Autodesk Inventor part; units mm, degrees
ref_plane "YZ Plane" through (0, 0, 0) normal (1, 0, 0) x (0, 1, 0)
ref_plane "XZ Plane" through (0, 0, 0) normal (0, 1, 0) x (-1, 0, 0)
ref_plane "XY Plane" through (0, 0, 0) normal (0, 0, 1) x (1, 0, 0)
sketch "Эскиз1" plane through (0, 0, 0) normal (0, 0, 1) x (1, 0, 0)
  line L0 (-54, -14) -> (54, -14)
  line L1 (54, -14) -> (54, 14)
  line L2 (54, 14) -> (-54, 14)
  line L3 (-54, 14) -> (-54, -14)
  line L4 (-54, -14) -> (54, 14) construction
  line L5 (54, -14) -> (-54, 14) construction
  point P0 (0, 0)
  dimension "d0" = 108
  dimension "d1" = 28
extrude "Выдавливание1" add sketch "Эскиз1" along normal blind 27.5
sketch "Эскиз2" plane through (0, 0, 27.5) normal (0, 0, 1) x (1, 0, 0)
  line L0 (-51, -11) -> (51, -11)
  line L1 (51, -11) -> (51, 11)
  line L2 (51, 11) -> (-51, 11)
  line L3 (-51, 11) -> (-51, -11)
  line L4 (-51, -11) -> (51, 11) construction
  line L5 (51, -11) -> (-51, 11) construction
  line L6 (54, 14) -> (-54, 14)
  line L7 (54, -14) -> (54, 14)
  point P0 (0, 0)
  dimension "d4" = 3
  dimension "d5" = 3
extrude "Выдавливание2" cut sketch "Эскиз2" against normal blind 24.5
sketch "Эскиз3" plane through (54, -14, 0) normal (1, 0, 0) x (0, 0, -1)
  line L0 (0, 28) -> (-27.5, 28)
  line L1 (0, 0) -> (-27.5, 0)
  line L2 (-27.5, 28) -> (-26, 28)
  line L3 (-26, 28) -> (-26, 0)
  line L4 (-26, 0) -> (-27.5, 0)
  line L5 (-27.5, 0) -> (-27.5, 28)
  point P0 (0, 14)
  dimension "d8" = 1.5
extrude "Выдавливание3" add sketch "Эскиз3" along normal blind 50
sketch "Эскиз4" plane through (0, 0, 27.5) normal (0, 0, 1) x (1, 0, 0)
  circle A0 centre (64, 0) radius 1.5
  line L0 (-54, -14) -> (104, -14)
  point P0 (0, 0)
  point P1 (54, -14)
  dimension "d11" = 3
  dimension "d12" = 14
  dimension "d13" = 10
extrude "Выдавливание4" cut sketch "Эскиз4" against normal blind 50
mirror "Зеркальное отражение1" about plane through (0, 0, 0) normal (1, 0, 0) of "Выдавливание3", "Выдавливание4"
properties part number "000.009 - Короб"
Model file for the job. Use its own axes, mm. A direction names the side the tool comes from. Round coordinates to 2 decimals unless told otherwise and drop trailing zeros. Order: outer loops, then holes, each group sorted by start corner. A loop starts at its lowest first (then second) coordinate and runs counter-clockwise, first axis right, second up.
(1) 3-axis set-ups, long thin cutter, end or side, ignore diameter. For faces 5 (the face through (1, 14, 14)), 6 (the face through (-1, -11, 15)), 7 (the face through (79, 0, 26)): which of +Z, -Z, +X, -X, +Y, -Y reach the whole face in a straight line?
(2) Band-saw the part on A-A (z = 18.5). List the corners of the cut face in (x, y).
(3) Pull direction X, two halves, no side cores. Call faces 1 (the face through (-54, 0, 13)), 2 (the face through (54, 0, 13)), 3 (the face through (-51, 0, 15)), 4 (the face through (-79, 0, 26)): released by +X, released by -X, zero draft, split by the parting line, or undercut.
(4) Band-saw the part on D-D (x = 73). List the corners of the cut face in (y, z).
(5) Drill centre lines: line 1 (Y direction, x = 35, z = 9.5); line 2 (X direction, y = 1.5, z = 17.5); line 3 (Y direction, x = 64, z = 26.85). Where is each one in solid material? Low to high.
(6) Band-saw the part on B-B (y = -8.25). List the corners of the cut face in (x, z).
(7) Band-saw the part on C-C (x = 20.5). List the corners of the cut face in (y, z).
(8) Pin check, flat tips, straight feed: pin 1 (8 mm diameter, centred on y = 5.5, z = 19.5, fed in from -X); pin 2 (3.5 mm diameter, centred on x = -64, y = 0, fed in from -Z); pin 3 (1 mm diameter, centred on y = 3.5, z = 5.5, fed in from +X). Stop position of each tip, or through.
Verdict:
1. face 5: +Z, -Z, +X, -X, +Y
1. face 6: +Z
1. face 7: -Z, +X, +Y, -Y
2. outline: (-54, -14) - (54, -14) - (54, 14) - (-54, 14) - close; hole (-51, -11) - (51, -11) - (51, 11) - (-51, 11) - close
3. face 1: released by -X
3. face 2: released by +X
3. face 3: undercut
3. face 4: zero draft
4. outline: (-14, 26) - (14, 26) - (14, 27.5) - (-14, 27.5) - close
5. line 1: y = -14 to -11, 11 to 14
5. line 2: x = -54 to -51, 51 to 54
5. line 3: y = -14 to -1.5, 1.5 to 14
6. outline: (-104, 26) - (-54, 26) - (-54, 0) - (54, 0) - (54, 26) - (104, 26) - (104, 27.5) - (51, 27.5) - (51, 3) - (-51, 3) - (-51, 27.5) - (-104, 27.5) - close
7. outline: (-14, 0) - (14, 0) - (14, 27.5) - (11, 27.5) - (11, 3) - (-11, 3) - (-11, 27.5) - (-14, 27.5) - close
8. pin 1: stops at x = -54
8. pin 2: stops at z = 26
8. pin 3: stops at x = 54
